Read the model definition and answer for the solid it produces. Units are mm, in the model's axes. A direction names the side the tool comes from. Coordinates: 2 decimals unless noted, no trailing zeros. Loops run counter-clockwise (first coordinate to the right, second up) from the corner with the lowest first, then second, coordinate; pieces in that order, holes last. Notation, with made-up numbers: (3.5, 76.25) - (21.5, 76.25) arc R25 cw to (21.5, 113.25) - close; hole circle Ø1 at (17.25, 34). An arc over 180 degrees is marked (long way). Use CSV: the item, a comma, the result in double quotes.
```python
from build123d import *

# Parameters (mm, degrees)
SKETCH_2_W          = 2
SKETCH_2_H          = 3
SKETCH_2_R          = 1.6
EXTRUDE_1_DEPTH     = 6
EXTRUDE_2_DEPTH     = 3
SKETCH_4_W          = 4
SKETCH_4_H          = 34.7
EXTRUDE_3_DEPTH     = 26
SKETCH_15_W         = 10
SKETCH_15_H         = 34.7
EXTRUDE_8_DEPTH     = 6
SKETCH_16_W         = 2
SKETCH_16_H         = 3
CUT_EXTRUDE_4_DEPTH = 6
CUT_EXTRUDE_5_DEPTH = 3
CUT_EXTRUDE_6_DEPTH = 3
SKETCH_20_W         = 8
SKETCH_20_H         = 5
EXTRUDE_9_DEPTH     = 40
SKETCH_22_R         = 1.5
CUT_EXTRUDE_7_DEPTH = 10
SKETCH_23_W         = 8
SKETCH_23_H         = 24
CUT_EXTRUDE_8_DEPTH = 10
FILLET_4_R          = 5
FILLET_5_R          = 2
FILLET_6_R          = 2
FILLET_7_R          = 2


with BuildPart() as part:
    # 草圖2 → 填料-伸長1 (new body)
    with BuildSketch(Plane(origin=(0, 0, 0), x_dir=(0, 0, -1), z_dir=(1, 0, 0))):
        with BuildLine():
            Line((13.55, 17.35), (-13.55, 17.35))
            Line((-13.55, 17.35), (-22.55, 17.35))
            Line((-22.55, 17.35), (-22.55, 6.1))
            ThreePointArc((-22.55, 6.1), (-16.45, 0), (-22.55, -6.1))
            Line((-22.55, -6.1), (-22.55, -17.35))
            Line((-22.55, -17.35), (-13.55, -17.35))
            Line((-13.55, -17.35), (13.55, -17.35))
            Line((13.55, -17.35), (13.55, 17.35))
        make_face()
        with Locations((-18.55, -12.85)):
            Rectangle(SKETCH_2_W, SKETCH_2_H, mode=Mode.SUBTRACT)
        with Locations((-10, -7.5)):
            Circle(SKETCH_2_R, mode=Mode.SUBTRACT)
        with Locations((10, -7.5)):
            Circle(SKETCH_2_R, mode=Mode.SUBTRACT)
        with Locations((-10, 7.5)):
            Circle(SKETCH_2_R, mode=Mode.SUBTRACT)
        with Locations((-18.55, 12.85)):
            Rectangle(SKETCH_2_W, SKETCH_2_H, mode=Mode.SUBTRACT)
        with Locations((10, 7.5)):
            Circle(SKETCH_2_R, mode=Mode.SUBTRACT)
    extrude(amount=EXTRUDE_1_DEPTH)

    # 草圖3 → 填料-伸長2 (add)
    with BuildSketch(Plane(origin=(6, 0, 0), x_dir=(0, 0, -1), z_dir=(1, 0, 0))):
        with BuildLine():
            Line((-13.55, 4.358898944), (-13.55, -4.358898944))
            ThreePointArc((-13.55, -4.358898944), (-17.239114454, -8.473163206), (-22.55, -10))
            Line((-22.55, -10), (-22.55, -8))
            ThreePointArc((-22.55, -8), (-14.55, 0), (-22.55, 8))
            Line((-22.55, 8), (-22.55, 10))
            ThreePointArc((-22.55, 10), (-17.239114454, 8.473163206), (-13.55, 4.358898944))
        make_face()
    extrude(amount=EXTRUDE_2_DEPTH)

    # 草圖4 → 填料-伸長3 (add)
    with BuildSketch(Plane.ZY):
        with Locations((-15.55, 0)):
            Rectangle(SKETCH_4_W, SKETCH_4_H)
    extrude(amount=-EXTRUDE_3_DEPTH)

    # 草圖15 → 填料-伸長8 (add)
    with BuildSketch(Plane(origin=(26, 0, 0), x_dir=(0, 0, -1), z_dir=(1, 0, 0))):
        with Locations((12.55, 0)):
            Rectangle(SKETCH_15_W, SKETCH_15_H)
    extrude(amount=EXTRUDE_8_DEPTH)

    # 草圖16 → 除料-伸長4 (cut)
    with BuildSketch(Plane(origin=(0, 0, -17.55), x_dir=(-1, 0, 0), z_dir=(0, 0, -1))):
        with Locations((-25, 7.85)):
            Rectangle(SKETCH_16_W, SKETCH_16_H)
        with Locations((-25, -7.85)):
            Rectangle(SKETCH_16_W, SKETCH_16_H)
    extrude(amount=-CUT_EXTRUDE_4_DEPTH, mode=Mode.SUBTRACT)

    # 草圖17 → 除料-伸長5 (cut)
    with BuildSketch(Plane(origin=(0, -9.35, 0), x_dir=(-1, 0, 0), z_dir=(0, -1, 0))):
        Polygon((-32, 17.55), (-31, 17.55), (-32, 16.55), align=None)
        Polygon((-32, 7.55), (-32, 8.55), (-31, 7.55), align=None)
    extrude(amount=-CUT_EXTRUDE_5_DEPTH, mode=Mode.SUBTRACT)

    # 草圖18 → 除料-伸長6 (cut)
    with BuildSketch(Plane(origin=(0, 9.35, 0), x_dir=(1, 0, 0), z_dir=(0, 1, 0))):
        Polygon((32, 17.55), (31, 17.55), (32, 16.55), align=None)
        Polygon((32, 7.55), (32, 8.55), (31, 7.55), align=None)
    extrude(amount=-CUT_EXTRUDE_6_DEPTH, mode=Mode.SUBTRACT)

    # 草圖20 → 填料-伸長9 (add)
    with BuildSketch(Plane(origin=(0, 17.35, 0), x_dir=(1, 0, 0), z_dir=(0, 1, 0))):
        with Locations((-4, -7.5)):
            Rectangle(SKETCH_20_W, SKETCH_20_H)
    extrude(amount=-EXTRUDE_9_DEPTH)

    # 草圖22 → 除料-伸長7 (cut)
    with BuildSketch(Plane.XY.offset(10)):
        with Locations((-4, 13.35)):
            Circle(SKETCH_22_R)
        with Locations((-4, -18.65)):
            Circle(SKETCH_22_R)
    extrude(amount=-CUT_EXTRUDE_7_DEPTH, mode=Mode.SUBTRACT)

    # 草圖23 → 除料-伸長8 (cut)
    with BuildSketch(Plane.XY.offset(10)):
        with Locations((-4, -2.65)):
            Rectangle(SKETCH_23_W, SKETCH_23_H)
    extrude(amount=-CUT_EXTRUDE_8_DEPTH, mode=Mode.SUBTRACT)

    # 圓角4
    fillet_4_edges = [part.edges().sort_by_distance(p)[0] for p in [
        (0, -14.65, 7.5),
    ]]
    fillet(fillet_4_edges, radius=FILLET_4_R)

    # 圓角5
    fillet_5_edges = [part.edges().sort_by_distance(p)[0] for p in [
        (0, -17.35, 7.5),
    ]]
    fillet(fillet_5_edges, radius=FILLET_5_R)

    # 圓角6
    fillet_6_edges = [part.edges().sort_by_distance(p)[0] for p in [
        (-8, -22.65, 7.5),
        (-8, 17.35, 7.5),
        (-8, -14.65, 7.5),
        (-8, 9.35, 7.5),
    ]]
    fillet(fillet_6_edges, radius=FILLET_6_R)

    # 圓角7
    fillet_7_edges = [part.edges().sort_by_distance(p)[0] for p in [
        (0, -22.65, 7.5),
    ]]
    fillet(fillet_7_edges, radius=FILLET_7_R)


solid = part.part
```
Q1. For a pull along X with two mould halves and no side action, classify faces 1 (the face through (3, -13, 17.55)), 2 (the face through (-0.6, -22.08, 7.46)), 3 (the face through (-7.43, -15.25, 7.46)), 4 (the face through (26, 0, -11)) as +X half, -X half, draft (parallel to the pull), parting line (faces both ways), or undercut.
Reported:
face 1,"draft"
face 2,"+X half"
face 3,"-X half"
face 4,"undercut"
Q2. A tool of negligible diameter and unlimited length cuts with its end or side. For faces 5 (the face through (3, 13, 19.55)), 6 (the face through (9, 0, 14)), 7 (the face through (25, -6.35, -16)), 8 (the face through (-1.43, -13.15, 7.46)), from which of +Z, -Z, +X, -X, +Y, -Y can it reach the whole face along a straight path? Write none if from no direction.
Reported:
face 5,"+X, -X"
face 6,"+Z, +X, +Y, -Y"
face 7,"+Z, -Z"
face 8,"+Z, -Z, -X"
Q3. The part is cut by section D-D on z = 3.5. Determine the outline of the cut face in (x, y).
Reported:
outline,"(0, -17.35) - (6, -17.35) - (6, 17.35) - (0, 17.35) - close"
Q4. The part is cut by section B-B on z = -10. Determine the outline of the cut face in (x, y).
Reported:
outline,"(0, -17.35) - (6, -17.35) - (6, -9.1) - (0, -9.1) - close; (0, -5.9) - (6, -5.9) - (6, 5.9) - (0, 5.9) - close; (0, 9.1) - (6, 9.1) - (6, 17.35) - (0, 17.35) - close; (26, -17.35) - (32, -17.35) - (32, 17.35) - (26, 17.35) - close"
Q5. Find the intervals of material crossed by probe 1 along Y at (x, z) = (4, 10); probe 2 along Z at (x, y) = (4, 7); probe 3 along Z at (x, y) = (1.5, 14), in increasing order. Write a range as [from, to].
Reported:
probe 1,"y = [-17.35, -9.1], [-5.9, 5.9], [9.1, 17.35]"
probe 2,"z = [-17.55, -11.52], [-8.48, 8.48], [11.52, 22.55]"
probe 3,"z = [-17.55, 17.55], [19.55, 22.55]"
Q6. The part is cut by section A-A on y = 0. Determine the outline of the cut face in (x, z), and give its area (3 significant figures).
Reported:
outline,"(0, -17.55) - (32, -17.55) - (32, -7.55) - (26, -7.55) - (26, -13.55) - (6, -13.55) - (6, 13.55) - (9, 13.55) - (9, 14.55) - (6, 14.55) - (6, 16.45) - (0, 16.45) - close"
area,"347 mm²"
Q7. Given P1, Ø9.5, axis at x = 11, z = -5, coming from the -Y side; P2, Ø2.5, axis at x = -4.5, y = 12, coming from the -Z side; P3, Ø6.5, axis at y = -1.5, z = 20, coming from the +X side; P4, Ø0.6, axis at x = 25, z = -15.5, coming from the -Y side, each flat-ended and moving along its own axis, determine where each tip first touches the part or whether it passes through.
Reported:
P1,"passes through"
P2,"stops at z = 5"
P3,"stops at x = 6"
P4,"stops at y = -17.35"
Q8. The part is cut by section C-C on y = -18.65. Determine the outline of the cut face in (x, z).
Reported:
outline,"(-8, 5) - (-5.5, 5) - (-5.5, 10) - (-8, 10) - close; (-2.5, 5) - (0.13, 5) - (0.13, 10) - (-2.5, 10) - close"
